The model under review builds one solid part; all positions refer to its coordinate system, in mm. A direction names the side the tool comes from. Round coordinates to 2 decimals unless told otherwise and drop trailing zeros. Loops run counter-clockwise (first coordinate to the right, second up) from the corner with the lowest first, then second, coordinate; pieces in that order, holes last. Notation, with made-up numbers: M 52.25,71 L 92.25,71 A26 ccw 92.25,105 Z; hole C 54,14.5 d3. An arc over 180 degrees is marked long. Answer in a Markdown table with one row per item. Add a question column.
Solid Edge part; units mm, degrees
sketch "Sketch1" plane through (0, 0, 0) normal (0, -1, 0) x (1, 0, 0)
  circle A0 centre (0, 0) radius 11.6
extrude "Protrusion1" add sketch "Sketch1" against normal blind 12
sketch "Sketch2" plane through (0, 0, 0) normal (0, -1, 0) x (1, 0, 0)
  circle A0 centre (0, 0) radius 5
extrude "Cutout1" cut sketch "Sketch2" against normal up to next
sketch "Sketch3" plane through (0, 0, 0) normal (1, 0, 0) x (0, 1, 0)
  line L0 (3, 11.6) -> (4.8065, 5.3)
  line L1 (4.8065, 5.3) -> (7.1935, 5.3)
  line L2 (7.1935, 5.3) -> (9, 11.6)
  line L3 (9, 11.6) -> (3, 11.6)
revolve "RevolvedCutout1" cut sketch "Sketch3" angle 360 about axis through (0, 0, 0) along (0, 1, 0)
properties material "Steel"
1. Take a section at B-B, the plane x = 0. State the section outline as (y, z) points, and give its area (3 significant figures).
2. To check wall thickness, follow probe 1 along Y at (x, z) = (0.75, 6); probe 2 along Y at (x, z) = (-6, -4.75); probe 3 along X at (y, z) = (9.5, -2.75). State the ranges of each line that lie inside material, in increasing order.
3. Take a section at A-A, the plane z = 0. State the section outline as (x, y) points.
4. Take a section at C-C, the plane y = 3.75. State the section outline as (x, z) points.
5. Mouldability with a two-part tool opening along Y and no side actions: class faces 3 (the conical face through (-5.646, 4.693, -0.741)), 4 (the cylindrical face through (-1.08, 5.92, -4.88)), 5 (the flat face through (-2, 0, -5)) as released by +Y, released by -Y, zero draft, split by the parting line, or undercut.
6. For pin 1 Ø2 at (x, y) = (-5, 2.5) entering from +Z; pin 2 Ø2 at (y, z) = (3.5, -8) entering from +X; pin 3 Ø9 at (x, z) = (0, 0) entering from -Y; pin 4 Ø2 at (y, z) = (3, -7) entering from +X, all flat-tipped, find the tip position at first contact; note any pin that passes through.
7. Machinability: for faces 1 (the cylindrical face through (-2.03, 6.017, 4.896)), 2 (the cylindrical face through (-11.59, 1.48, 0.51)), which of the approach directions +Z, -Z, +X, -X, +Y, -Y give a long, thin tool a straight path to every point of the face, cutting with its end or side? Answer none if there is none.
Check sheet entries:
| question | item | result |
|---|---|---|
| 1 | outline | M 0,-11.6 L 3,-11.6 L 4.81,-5.3 L 7.19,-5.3 L 9,-11.6 L 12,-11.6 L 12,-5 L 0,-5 Z; M 0,5 L 12,5 L 12,11.6 L 9,11.6 L 7.19,5.3 L 4.81,5.3 L 3,11.6 L 0,11.6 Z |
| 1 | area | 106 mm^2 |
| 2 | probe 1 | y = 0 to 4.59, 7.41 to 12 |
| 2 | probe 2 | y = 0 to 4.13, 7.87 to 12 |
| 2 | probe 3 | x = -11.27 to -4.18, 4.18 to 11.27 |
| 3 | outline | M -11.6,0 L -5,0 L -5,12 L -11.6,12 L -11.6,9 L -5.3,7.19 L -5.3,4.81 L -11.6,3 Z; M 5,0 L 11.6,0 L 11.6,3 L 5.3,4.81 L 5.3,7.19 L 11.6,9 L 11.6,12 L 5,12 Z |
| 4 | outline | C 0,0 d17.97; hole C 0,0 d10 |
| 5 | face 3 | undercut |
| 5 | face 4 | zero draft |
| 5 | face 5 | released by -Y |
| 6 | pin 1 | stops at z = 10.89 |
| 6 | pin 2 | stops at x = 9.15 |
| 6 | pin 3 | passes through |
| 6 | pin 4 | stops at x = 9.93 |
| 7 | face 1 | none |
| 7 | face 2 | +Y, -Y |
